from build123d import *

# Parameters (mm, degrees)
SKETCH1_R               = 8.255
BOSS_EXTRUDE1_DEPTH     = 12.7
SKETCH6_W               = 0.635
SKETCH6_H               = 14.1852904
CUT_EXTRUDE3_DEPTH      = 12.7
CUT_EXTRUDE3_DEPTH_BACK = 12.7


with BuildPart() as part:
    # Sketch1 → Boss-Extrude1 (new body)
    with BuildSketch(Plane(origin=(0, 0, 0), x_dir=(1, 0, 0), z_dir=(0, 1, 0))):
        with Locations((4.445, 5.08)):
            Circle(SKETCH1_R)
        Polygon((4.445, 0), (9.525, 0), (9.525, 10.16), (-0.635, 10.16), (-0.635, 0), align=None, mode=Mode.SUBTRACT)
    extrude(amount=BOSS_EXTRUDE1_DEPTH)

    # Sketch5 → Revolve4 (revolve)
    with BuildSketch(Plane(origin=(0, 0, -5.08), x_dir=(-1, 0, 0), z_dir=(0, 0, -1))):
        Polygon((-12.7, 12.7), (-4.445, 12.7), (-4.445, 20.246092455), (-4.445, 36.336009477), (-7.62, 36.336009477), (-7.62, 22.150719077), align=None)
    revolve(axis=Axis((4.445, 36.336009477, -5.08), (0, 1, 0)))

    # Sketch6 → Cut-Extrude3 (cut, two sides)
    with BuildSketch(Plane(origin=(0, 0, -5.08), x_dir=(-1, 0, 0), z_dir=(0, 0, -1))) as cut_extrude3_sk:
        with Locations((-7.3025, 29.243364277)):
            Rectangle(SKETCH6_W, SKETCH6_H)
    extrude(amount=CUT_EXTRUDE3_DEPTH, mode=Mode.SUBTRACT)
    extrude(cut_extrude3_sk.sketch, amount=-CUT_EXTRUDE3_DEPTH_BACK, mode=Mode.SUBTRACT)


solid = part.part
Model file for the job. Use its own axes, mm. A direction names the side the tool comes from. Give positions to 0.01 mm unless a question says otherwise; leave off trailing zeros. Write each loop counter-clockwise with the first axis right and the second up, starting at its lowest first coordinate (ties: lowest second). Pieces come first, ordered by that corner, then holes. Notation, with made-up numbers: (50, 15.5) - (88, 15.5) arc R24 ccw to (88, 46.5) - close; hole circle Ø2 at (60.5, 11.25). An arc over 180 degrees is marked (long way). Answer as CSV lines item,"result".
1. Band-saw the part on C-C (y = 29). Write the cut outline in (x, z) (3 decimals), and give its area (3 significant figures).
Responses:
outline,"(6.985, -6.985) - (6.985, -3.175) arc R3.175 ccw (long way) to start"
area,"30.0 mm2"
2. Drill centre lines: L1, parallel to Z at x = 7.25, y = 12; L2, parallel to Z at x = 2, y = 7; L3, parallel to X at y = 14.5, z = -10.5. Where is each one in solid material? Low to high. Write a range as [from, to].
Responses:
L1,"z = [-12.84, -10.16], [0, 2.68]"
L2,"z = [-12.96, -10.16], [0, 2.8]"
L3,"x = [-0.43, 9.32]"
3. Pin check, flat tips, straight feed: pin 1 (1.5 mm diameter, centred on y = 9, z = -1, fed in from +X); pin 2 (8 mm diameter, centred on x = 8, y = 24.5, fed in from +Z); pin 3 (1.9 mm diameter, centred on y = 28, z = -5, fed in from +X) (3 decimals); pin 4 (1.5 mm diameter, centred on x = -1, y = 21.5, fed in from +Z). Stop position of each tip, or through.
Responses:
pin 1,"stops at x = 12"
pin 2,"stops at z = -1.63"
pin 3,"stops at x = 6.985"
pin 4,"passes through"
4. Band-saw the part on D-D (y = 21.5). Write the cut outline in (x, z) (3 decimals).
Responses:
outline,"circle Ø7.05 at (4.445, -5.08)"
5. Band-saw the part on B-B (z = -5.08). Write the cut outline in (x, y) (3 decimals), and give its area (3 significant figures).
Responses:
outline,"(-3.81, 0) - (-0.635, 0) - (-0.635, 12.7) - (9.525, 12.7) - (9.525, 0) - (12.7, 0) - (12.7, 12.7) - (7.62, 22.151) - (6.985, 22.151) - (6.985, 36.336) - (1.27, 36.336) - (1.27, 22.151) - (-3.81, 12.7) - close"
area,"270 mm2"
6. Band-saw the part on A-A (y = 6). Write the cut outline in (x, z) (3 decimals), and give its area (3 significant figures).
Responses:
outline,"circle Ø16.51 at (4.445, -5.08); hole (-0.635, -10.16) - (9.525, -10.16) - (9.525, 0) - (-0.635, 0) - close"
area,"111 mm2"
7. Two-plate mould, pull along Z, no slides. Class faces 5 (the face through (4, 36.336, -5)), 6 (the face through (3.4, 19.5, -0.6)), 7 (the face through (4, 12.7, -5)): +Z half, -Z half, draft (parallel to the pull), parting line (faces both ways), or undercut.
Responses:
face 5,"draft"
face 6,"parting line"
face 7,"undercut"
8. 3-axis set-ups, long thin cutter, end or side, ignore diameter. For faces 1 (the face through (-0.635, 6, -5)), 2 (the face through (1.27, 29.14, -5.19)), 3 (the face through (2.66, 6.26, 2.98)), 4 (the face through (6.985, 29, -5)): which of +Z, -Z, +X, -X, +Y, -Y reach the whole face in a straight line?
Responses:
face 1,"-Y"
face 2,"+Y"
face 3,"+Y, -Y"
face 4,"+Z, -Z, +X, +Y"
